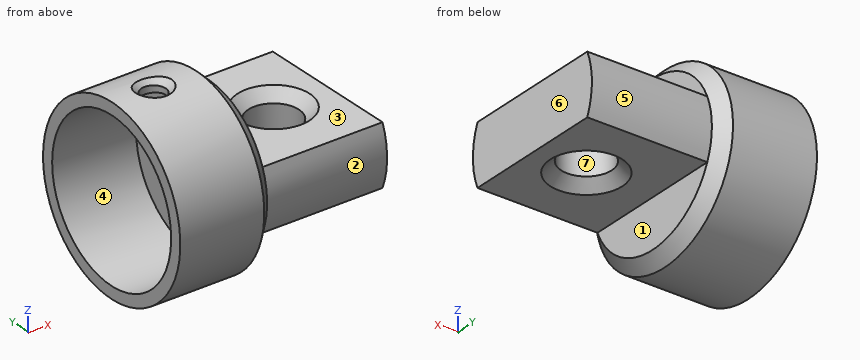
from build123d import *

# Parameters (mm, degrees)
F0_R            = 7.5
F1_DEPTH        = 8
F2_T            = -1
F3_SIZE         = 1
F5_DEPTH        = 10
F8_D            = 4.2
F8_DEPTH        = 2.5
F8_CSINK_D      = 6
F8_CSINK_ANGLE  = 90
F11_D           = 4.2
F11_DEPTH       = 2.5
F11_CSINK_D     = 6
F11_CSINK_ANGLE = 90
F15_D           = 2
F15_DEPTH       = 2.5
F15_CSINK_D     = 3
F15_CSINK_ANGLE = 90


with BuildPart() as f1:
    # F0 (on Right) → F1 (new body)
    with BuildSketch(Plane.YZ):
        Circle(F0_R)
    extrude(amount=F1_DEPTH)

    # F2
    f2_openings = [f1.faces().sort_by_distance(p)[0] for p in [
        (0, 0, 0),
    ]]
    offset(amount=F2_T, openings=f2_openings)

    # F3
    f3_edges = [f1.edges().sort_by_distance(p)[0] for p in [
        (8, -7.5, 0),
    ]]
    chamfer(f3_edges, length=F3_SIZE)

    # F4 (on face) → F5 (join)
    with BuildSketch(Plane.YZ.offset(8)):
        with BuildLine():
            Line((-6, -2.5), (0, -2.5))
            Line((0, -2.5), (6, -2.5))
            ThreePointArc((6, -2.5), (6.5, 0), (6, 2.5))
            Line((6, 2.5), (0, 2.5))
            Line((0, 2.5), (-6, 2.5))
            ThreePointArc((-6, 2.5), (-6.5, 0), (-6, -2.5))
        make_face()
    extrude(amount=F5_DEPTH)

    # F8
    with Locations(Plane.XY.offset(2.5)):
        with Locations((13.5, 0)):
            CounterSinkHole(F8_D / 2, F8_CSINK_D / 2, depth=F8_DEPTH, counter_sink_angle=F8_CSINK_ANGLE)

    # F11
    with Locations(Plane(origin=(0, 0, -2.5), x_dir=(1, 0, 0), z_dir=(0, 0, -1))):
        with Locations((13.5, 0)):
            CounterSinkHole(F11_D / 2, F11_CSINK_D / 2, depth=F11_DEPTH, counter_sink_angle=F11_CSINK_ANGLE)

    # F15
    with Locations(Plane.XY.offset(7.5)):
        with Locations((3.5, 0)):
            CounterSinkHole(F15_D / 2, F15_CSINK_D / 2, depth=F15_DEPTH, counter_sink_angle=F15_CSINK_ANGLE)


solid = f1.part
For this review, take the finished solid that the model builds, in its own axes (mm). Face numbers are marked on the shaded views. A direction names the side the tool comes from. Coordinates: 2 decimals unless noted, no trailing zeros. Order: outer loops, then holes, each group sorted by start corner. A loop starts at its lowest first (then second) coordinate and runs counter-clockwise, first axis right, second up. Notation, with made-up numbers: (24, 75.25) -> (42, 75.25) arc R28 ccw to (42, 94.25) -> close; hole circle Ø10 at (7, 19.5). An arc over 180 degrees is marked (long way). Return JSON: item names as keys, results as strings.
1. For line 1 (X direction, y = 0, z = 0.4); line 2 (X direction, y = 2, z = 3.25); line 3 (X direction, y = 4.75, z = 2), list the stretches that pass through material, from the lowest coordinate up. Write a range as from..to.
Answer block:
{"line 1": "7..11.4, 15.6..18", "line 2": "7..8", "line 3": "7..18"}
2. The part is to be moulded in two halves that separate along X. For the marked faces 5, 6 and 7, say which applies: +X half, -X half, draft (parallel to the pull), parting line (faces both ways), or undercut.
Answer block:
{"face 5": "draft", "face 6": "+X half", "face 7": "undercut"}
3. We need section A-A on x = 13.5. Write out the cut boundary in (y, z), and give its area (3 significant figures).
Answer block:
{"outline": "(-6, -2.5) -> (-3, -2.5) -> (-2.1, -1.6) -> (-2.1, 1.6) -> (-3, 2.5) -> (-6, 2.5) arc R6.5 ccw to start; (2.1, -1.6) -> (3, -2.5) -> (6, -2.5) arc R6.5 ccw to (6, 2.5) -> (3, 2.5) -> (2.1, 1.6) -> close", "area": "40.7 mm²"}
4. We need section B-B on y = 0. Write out the cut boundary in (x, z).
Answer block:
{"outline": "(0, -7.5) -> (7, -7.5) -> (8, -6.5) -> (8, -2.5) -> (10.5, -2.5) -> (11.4, -1.6) -> (11.4, 1.6) -> (10.5, 2.5) -> (8, 2.5) -> (8, 6.5) -> (7, 7.5) -> (5, 7.5) -> (4.5, 7) -> (4.5, 6.5) -> (7, 6.5) -> (7, -6.5) -> (0, -6.5) -> close; (0, 6.5) -> (2.5, 6.5) -> (2.5, 7) -> (2, 7.5) -> (0, 7.5) -> close; (15.6, -1.6) -> (16.5, -2.5) -> (18, -2.5) -> (18, 2.5) -> (16.5, 2.5) -> (15.6, 1.6) -> close"}
5. We need section D-D on x = 6. Write out the cut boundary in (y, z).
Answer block:
{"outline": "circle Ø15 at (0, 0); hole circle Ø13 at (0, 0)"}
6. For pin 1 Ø1.5 at (x, z) = (5.5, -3) entering from +Y; pin 2 Ø1.2 at (y, z) = (-3, 5) entering from +X; pin 3 Ø5 at (x, y) = (12.5, -2.5) entering from +Z, all flat-tipped, find the tip position at first contact; note any pin that passes through.
Answer block:
{"pin 1": "y = 7.15", "pin 2": "x = 8", "pin 3": "z = 2.5"}
7. Machinability: for the marked faces 1, 2, 3 and 4, which of the approach directions +Z, -Z, +X, -X, +Y, -Y give a long, thin tool a straight path to every point of the face, cutting with its end or side? Answer none if there is none.
Answer block:
{"face 1": "-Z, +X, +Y, -Y", "face 2": "+X, -Y", "face 3": "+Z, +X, +Y, -Y", "face 4": "-X"}
8. We need section C-C on z = 0. Write out the cut boundary in (x, y), and give its area (3 significant figures).
Answer block:
{"outline": "(0, -7.5) -> (7, -7.5) -> (8, -6.5) -> (18, -6.5) -> (18, 6.5) -> (8, 6.5) -> (7, 7.5) -> (0, 7.5) -> (0, 6.5) -> (7, 6.5) -> (7, -6.5) -> (0, -6.5) -> close; hole circle Ø4.2 at (13.5, 0)", "area": "144 mm²"}
